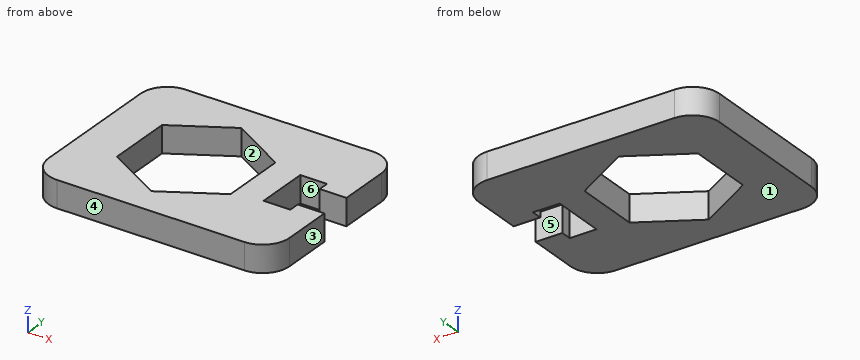
```python
from build123d import *

# Parameters (mm, degrees)
BOSS_EXTRU_1_DEPTH = 2.5
CONG_1_R           = 5


with BuildPart() as part:
    # Esquisse1 → Boss.-Extru.1 (new body, symmetric)
    with BuildSketch(Plane.XY):
        Polygon((22.5, 3), (22.5, 17.5), (-22.5, 17.5), (-22.5, -17.5), (22.5, -17.5), (22.5, -3), (17.5, -3), (17.5, -5), (12.5, -5), (12.5, 5), (17.5, 5), (17.5, 3), align=None)
        Polygon((7.1, 6.119912853), (-3.5, 12.239825707), (-14.1, 6.119912853), (-14.1, -6.119912853), (-3.5, -12.239825707), (7.1, -6.119912853), align=None, mode=Mode.SUBTRACT)
    extrude(amount=BOSS_EXTRU_1_DEPTH, both=True)

    # Congé1
    cong_1_edges = [part.edges().sort_by_distance(p)[0] for p in [
        (-22.5, 17.5, 0),
        (22.5, 17.5, 0),
        (22.5, -17.5, 0),
        (-22.5, -17.5, 0),
    ]]
    fillet(cong_1_edges, radius=CONG_1_R)


solid = part.part
```
Source: CAD feature listing. Evaluate the final solid. Frame: model axes, mm. Face numbers are marked on the shaded views. A direction names the side the tool comes from. Round coordinates to 2 decimals unless told otherwise and drop trailing zeros. Loops run counter-clockwise (first coordinate to the right, second up) from the corner with the lowest first, then second, coordinate; pieces in that order, holes last. Notation, with made-up numbers: M 33,39.25 L 81,39.25 A28 cw 81,61.25 Z; hole C 64,8.5 d4. An arc over 180 degrees is marked long. Put each result on its own line as item: value.
(1) Section C-C, the plane x = -3. Return loops of the section in (y, z).
Solutions:
outline: M -17.5,-2.5 L -11.95,-2.5 L -11.95,2.5 L -17.5,2.5 Z; M 11.95,-2.5 L 17.5,-2.5 L 17.5,2.5 L 11.95,2.5 Z
(2) Pull-direction query (X, two-part tool) for the marked faces 1, 2 and 3; classes: released by +X, released by -X, zero draft, split by the parting line, or undercut.
Solutions:
face 1: zero draft
face 2: undercut
face 3: released by +X
(3) First-contact query: pin 1 (2.5 mm diameter, centred on y = -1, z = 0, fed in from +X); pin 2 (1.5 mm diameter, centred on x = 21, z = 0.5, fed in from +Y). Flat tips, straight axial feed; report the tip coordinate or a pass-through.
Solutions:
pin 1: x = 12.5
pin 2: y = 16.68
(4) Section B-B, the plane z = -1.6. Return loops of the section in (x, y).
Solutions:
outline: M -22.5,-12.5 A5 ccw -17.5,-17.5 L 17.5,-17.5 A5 ccw 22.5,-12.5 L 22.5,-3 L 17.5,-3 L 17.5,-5 L 12.5,-5 L 12.5,5 L 17.5,5 L 17.5,3 L 22.5,3 L 22.5,12.5 A5 ccw 17.5,17.5 L -17.5,17.5 A5 ccw -22.5,12.5 Z; hole M -14.1,-6.12 L -3.5,-12.24 L 7.1,-6.12 L 7.1,6.12 L -3.5,12.24 L -14.1,6.12 Z
(5) Section A-A, the plane y = -1.5. Return loops of the section in (x, z), and give its area (3 significant figures).
Solutions:
outline: M -22.5,-2.5 L -14.1,-2.5 L -14.1,2.5 L -22.5,2.5 Z; M 7.1,-2.5 L 12.5,-2.5 L 12.5,2.5 L 7.1,2.5 Z
area: 69.0 mm²
(6) Ray query, line 1 (X direction, y = 1, z = 1.9); line 2 (Y direction, x = 13.5, z = 1.8); line 3 (X direction, y = 6, z = 2.25). Return the intervals inside material, ascending. Write a range as [from, to].
Solutions:
line 1: [-22.5, -14.1], [7.1, 12.5]
line 2: [-17.5, -5], [5, 17.5]
line 3: [-22.5, -14.1], [7.1, 22.5]
(7) Access query for the marked faces 4, 5 and 6. Directions: +Z, -Z, +X, -X, +Y, -Y. A direction counts if a zero-diameter tool reaches every point of the face in a straight line with its end or side. Return the directions, or none.
Solutions:
face 4: +Z, -Z, +X, -X, -Y
face 5: +Z, -Z, +X
face 6: +Z, -Z
